from build123d import *

# Parameters (mm, degrees)
BOX_W          = 100
BOX_H          = 100
BOX_DEPTH      = 10
CYLINDER_R     = 25
CYLINDER_DEPTH = 10
BOX001_W       = 60
BOX001_H       = 60
BOX001_DEPTH   = 10
FILLET_R       = 15


with BuildPart() as cube:
    # Box → Box (new body)
    with BuildSketch(Plane.XY):
        with Locations((50, 50)):
            Rectangle(BOX_W, BOX_H)
    extrude(amount=BOX_DEPTH)


with BuildPart() as cylinder:
    # Cylinder → Cylinder (new body)
    with BuildSketch(Plane(origin=(50, 50, 10), x_dir=(1, 0, 0), z_dir=(0, 0, 1))):
        Circle(CYLINDER_R)
    extrude(amount=CYLINDER_DEPTH)


with BuildPart() as model_fusion:
    # Box001 → Box001 (new body)
    with BuildSketch(Plane(origin=(20, 20, 10), x_dir=(1, 0, 0), z_dir=(0, 0, 1))):
        with Locations((30, 30)):
            Rectangle(BOX001_W, BOX001_H)
    extrude(amount=BOX001_DEPTH)

    # Fillet
    fillet_edges = [model_fusion.edges().sort_by_distance(p)[0] for p in [
        (20, 20, 15),
        (20, 80, 15),
    ]]
    fillet(fillet_edges, radius=FILLET_R)

    # Cut: cut Cylinder
    add(cylinder.part, mode=Mode.SUBTRACT)

    # Fusion: union Cube
    add(cube.part)


solid = model_fusion.part
Work out the finished part from the listing and answer in its coordinate system (mm). A direction names the side the tool comes from. Give positions to 0.01 mm unless a question says otherwise; leave off trailing zeros. Order: outer loops, then holes, each group sorted by start corner. A loop starts at its lowest first (then second) coordinate and runs counter-clockwise, first axis right, second up. Notation, with made-up numbers: M -11.5,4 L 22.5,4 A10 cw 22.5,11 Z; hole C 33,28.25 d7. An arc over 180 degrees is marked long. Return JSON: item names as keys, results as strings.
Q1. Find the intervals of material crossed by line 1 along Y through (x, z) = (50, 16.5); line 2 along Z through (x, y) = (73.5, 52); line 3 along Y through (x, z) = (43, 16.75), in increasing order. Write a range as [from, to].
Answer below:
{"line 1": "y = [20, 25], [75, 80]", "line 2": "z = [0, 10]", "line 3": "y = [20, 26], [74, 80]"}
Q2. Find section D-D, the plane x = 11. Write down the section's boundary in (y, z).
Answer below:
{"outline": "M 0,0 L 100,0 L 100,10 L 0,10 Z"}
Q3. Find section A-A, the plane z = 17.25. Write down the section's boundary in (x, y).
Answer below:
{"outline": "M 20,35 A15 ccw 35,20 L 80,20 L 80,80 L 35,80 A15 ccw 20,65 Z; hole C 50,50 d50"}
Q4. Which of the six approach directions +Z, -Z, +X, -X, +Y, -Y give full straight-line access (tool end or side, diameter ignored) to faces 1 (the face through (24.28, 75.49, 15.07)), 2 (the face through (20, 50, 15)), 3 (the face through (57, 20, 15)), 4 (the face through (57, 80, 15)), 5 (the face through (80, 50, 15))?
Answer below:
{"face 1": "+Z, -X, +Y", "face 2": "+Z, -X, +Y, -Y", "face 3": "+Z, +X, -X, -Y", "face 4": "+Z, +X, -X, +Y", "face 5": "+Z, +X, +Y, -Y"}
Q5. Find section B-B, the plane x = 50. Write down the section's boundary in (y, z).
Answer below:
{"outline": "M 0,0 L 100,0 L 100,10 L 80,10 L 80,20 L 75,20 L 75,10 L 25,10 L 25,20 L 20,20 L 20,10 L 0,10 Z"}
Q6. The mould has two halves that part along X. Classify faces 6 (the face through (49, 0, 5)), 7 (the face through (0, 49, 5)), 8 (the face through (30, 35, 15)): pulls with the +X half, pulls with the -X half, needs draft (parallel to the pull), parting line crosses it, or undercut.
Answer below:
{"face 6": "needs draft", "face 7": "pulls with the -X half", "face 8": "undercut"}
Q7. Each of these flat-tipped pins is pushed along its axis until it touches: pin 1 (1 mm diameter, centred on y = 12.5, z = 6.5, fed in from -X); pin 2 (5 mm diameter, centred on y = 56, z = 17, fed in from +X); pin 3 (5 mm diameter, centred on y = 65, z = 13, fed in from -X); pin 4 (1 mm diameter, centred on x = 31, z = 16.5, fed in from +Y). Where does it stop, or does it pass through?
Answer below:
{"pin 1": "stops at x = 0", "pin 2": "stops at x = 80", "pin 3": "stops at x = 20", "pin 4": "stops at y = 79.59"}
